```python
from build123d import *

# Parameters (mm, degrees)
F2_R      = 1.15
F2_R_2    = 1
F2_R_3    = 0.55
F2_R_4    = 0.8
F2_R_5    = 0.85
F2_R_6    = 0.5
F2_R_7    = 0.675
F3_DEPTH  = 6.501
F4_R      = 1
F5_R      = 0.2
F6_SIZE   = 0.2
F8_DEPTH  = 0.5
F9_R      = 0.675
F10_DEPTH = 10.701
F11_R     = 0.9
F11_R_2   = 0.675
F12_DEPTH = 1.2


with BuildPart() as f1:
    # F0 (on Front) → F1 (revolve)
    with BuildSketch(Plane.XZ):
        Polygon((3.25, 5.2), (3.25, 0), (6.5, 0), (6.5, 4.7), (21.4, 4.7), (21.4, 6.7), (4, 6.7), (4, 7.5), (3, 7.5), (3, 8.35), (4, 8.35), (4, 11.2), (1.5, 11.2), (1.5, 5.2), align=None)
    revolve(axis=Axis((0, 0, 5.6), (0, 0, 1)))

    # F2 (on face) → F3 (cut, through all)
    with BuildSketch(Plane(origin=(0, 0, 4.7), x_dir=(1, 0, 0), z_dir=(0, 0, -1))):
        with Locations((19.5, 0)):
            Circle(F2_R)
        with Locations((18.3240061053, -6.6693927949)):
            Circle(F2_R)
        with Locations((14.9378666408, -12.5343583889)):
            Circle(F2_R)
        with Locations((9.75, -16.8874953738)):
            Circle(F2_R)
        with Locations((3.3861394645, -19.2037511837)):
            Circle(F2_R)
        with Locations((-3.3861394645, -19.2037511837)):
            Circle(F2_R)
        with Locations((-9.75, -16.8874953738)):
            Circle(F2_R)
        with Locations((-14.9378666408, -12.5343583889)):
            Circle(F2_R)
        with Locations((-17.8541597949, -6.4983827232)):
            Circle(F2_R_2)
        with Locations((11.6913429511, 6.75)):
            Circle(F2_R_2)
        with Locations((8.6776327308, 10.3415999821)):
            Circle(F2_R_2)
        with Locations((12.6858503806, -4.6172719349)):
            Circle(F2_R_2)
        with Locations((13.5, 0)):
            Circle(F2_R_2)
        with Locations((10.3415999821, -8.6776327308)):
            Circle(F2_R_2)
        with Locations((6.75, -11.6913429511)):
            Circle(F2_R_2)
        with Locations((2.3442503985, -13.2949046657)):
            Circle(F2_R_2)
        with Locations((-2.3442503985, -13.2949046657)):
            Circle(F2_R_2)
        with Locations((-6.75, -11.6913429511)):
            Circle(F2_R_2)
        with Locations((-10.3415999821, -8.6776327308)):
            Circle(F2_R_2)
        with Locations((-12.6858503806, -4.6172719349)):
            Circle(F2_R_2)
        with Locations((-13.5, 0)):
            Circle(F2_R_2)
        with Locations((-12.6858503806, 4.6172719349)):
            Circle(F2_R_2)
        with Locations((-8.6776327308, 10.3415999821)):
            Circle(F2_R_2)
        with Locations((-4.6172719349, 12.6858503806)):
            Circle(F2_R_2)
        with Locations((0, 13.5)):
            Circle(F2_R_2)
        with Locations((4.6172719349, 12.6858503806)):
            Circle(F2_R_2)
        with Locations((18.7113473072, -3.2993153757)):
            Circle(F2_R_3)
        with Locations((12.212964584, -14.5548444193)):
            Circle(F2_R_3)
        with Locations((0, -19)):
            Circle(F2_R_3)
        with Locations((-12.212964584, -14.5548444193)):
            Circle(F2_R_3)
        with Locations((6.4983827232, -17.8541597949)):
            Circle(F2_R_4)
        with Locations((17.6164932368, 7.1175252749)):
            Circle(F2_R_2)
        with Locations((13.5, 11.2)):
            Circle(F2_R_5)
        with Locations((11.1842488695, 9.3846991014)):
            Circle(F2_R_6)
        with Locations((-6.4983827232, 17.8541597949)):
            Circle(F2_R_4)
        with Locations((-12.7134815208, 14.1197516841)):
            Circle(F2_R_2)
        with Locations((-17.2341356777, 3.0388431092)):
            Circle(F2_R_7)
        with Locations((-14.3341356777, 2.5274948651)):
            Circle(F2_R_6)
        with BuildLine():
            Line((6.1356301693, 20.5015619509), (5.7498180769, 19.3141544258))
            ThreePointArc((5.7498180769, 19.3141544258), (5.4850516502, 16.8812531642), (6.7008745932, 19.0051374314))
            Line((6.7008745932, 19.0051374314), (7.0866866856, 20.1925449565))
            ThreePointArc((7.0866866856, 20.1925449565), (6.6129636796, 20.3526094487), (6.1356301693, 20.5015619509))
        make_face()
    extrude(amount=-F3_DEPTH, mode=Mode.SUBTRACT)

    # F4
    f4_edges = [f1.edges().sort_by_distance(p)[0] for p in [
        (-6.5, 0, 4.7),
    ]]
    fillet(f4_edges, radius=F4_R)

    # F5
    f5_edges = [f1.edges().sort_by_distance(p)[0] for p in [
        (-4, 0, 6.7),
    ]]
    fillet(f5_edges, radius=F5_R)

    # F6
    f6_edges = [f1.edges().sort_by_distance(p)[0] for p in [
        (-4, 0, 11.2),
    ]]
    chamfer(f6_edges, length=F6_SIZE)

    # F7 (on face) → F8 (cut)
    with BuildSketch(Plane(origin=(0, 0, 0), x_dir=(1, 0, 0), z_dir=(0, 0, -1))):
        with BuildLine():
            ThreePointArc((-5.8896094947, 2.75), (-6.5, 0), (-5.8896094947, -2.75))
            Line((-5.8896094947, -2.75), (-1.7320508076, -2.75))
            ThreePointArc((-1.7320508076, -2.75), (-3.25, 0), (-1.7320508076, 2.75))
            Line((-1.7320508076, 2.75), (-5.8896094947, 2.75))
        make_face()
        with BuildLine():
            Line((1.7320508076, -2.75), (5.8896094947, -2.75))
            ThreePointArc((5.8896094947, -2.75), (6.3455678121, -1.4084633976), (6.5, 0))
            ThreePointArc((6.5, 0), (6.3455678121, 1.4084633976), (5.8896094947, 2.75))
            Line((5.8896094947, 2.75), (1.7320508076, 2.75))
            ThreePointArc((1.7320508076, 2.75), (2.8453176558, 1.5705627774), (3.25, 0))
            ThreePointArc((3.25, 0), (2.8453176558, -1.5705627774), (1.7320508076, -2.75))
        make_face()
    extrude(amount=-F8_DEPTH, mode=Mode.SUBTRACT)

    # F9 (on face) → F10 (cut, through all)
    with BuildSketch(Plane(origin=(0, 0, 0.5), x_dir=(1, 0, 0), z_dir=(0, 0, -1))):
        with Locations((-4.9, 0)):
            Circle(F9_R)
    extrude(amount=-F10_DEPTH, mode=Mode.SUBTRACT)

    # F11 (on face) → F12 (cut)
    with BuildSketch(Plane(origin=(0, 0, 0.5), x_dir=(1, 0, 0), z_dir=(0, 0, -1))):
        with Locations((-4.9, 0)):
            Circle(F11_R)
        with Locations((-4.9, 0)):
            Circle(F11_R_2, mode=Mode.SUBTRACT)
        with Locations((-4.9, 0)):
            Circle(F11_R_2)
    extrude(amount=-F12_DEPTH, mode=Mode.SUBTRACT)


solid = f1.part
```
CAD build for the part. Positions are in the model's coordinates, mm. A direction names the side the tool comes from. Round coordinates to 2 decimals unless told otherwise and drop trailing zeros. Answer as CSV lines item,"result". Start each with the question number.
1. Pull direction X, two halves, no side cores. Call faces 3 (the face through (18.16, 3.28, 5.69)), 4 (the face through (5, 0, 0.5)): +X half, -X half, draft (parallel to the pull), parting line (faces both ways), or undercut.
2. Tool access for faces 1 (the face through (-4.256, -0.203, 4.165)), 2 (the face through (1.5, -2.883, 2.564)): list every direction of +Z, -Z, +X, -X, +Y, -Y with a clear straight run to the whole face (end or side of a thin tool).
3. Drill centre lines: L1, parallel to Y at x = -13.5, z = 5.6; L2, parallel to X at y = -7, z = 6.25; L3, parallel to Y at x = 13.5, z = 5.95. Where is each one in solid material? Low to high. Write a range as [from, to].
4. Saw through at A-A, the plane x = 0. Count the separate pieces of the cut face and the enclosed holes in it, and give its area (3 significant figures).
5. Pin check, flat tips, straight feed: pin 1 (2.5 mm diameter, centred on x = 6.75, y = 11.69, fed in from +Z); pin 2 (2 mm diameter, centred on x = -4.9, y = 0, fed in from -Z); pin 3 (13 mm diameter, centred on x = 0, y = -4.5, fed in from -Z); pin 4 (6 mm diameter, centred on x = 9, z = 7, fed in from -Y). Stop position of each tip, or through.
Model answer:
1,face 3,"undercut"
1,face 4,"draft"
2,face 1,"+Z, -Z"
2,face 2,"-Z"
3,L1,"y = [-16.6, -14.74], [-13.5, -5.2], [-4.04, -1], [1, 4.04], [5.2, 16.6]"
3,L2,"x = [-20.22, 10.72], [12.66, 16.62], [18.61, 20.22]"
3,L3,"y = [-16.6, -12.05], [-10.35, -1], [1, 4.04], [5.2, 16.6]"
4,separate pieces,"4"
4,enclosed holes,"0"
4,area,"123 mm²"
5,pin 1,"stops at z = 6.7"
5,pin 2,"stops at z = 0.5"
5,pin 3,"stops at z = 0"
5,pin 4,"stops at y = -20.54"
